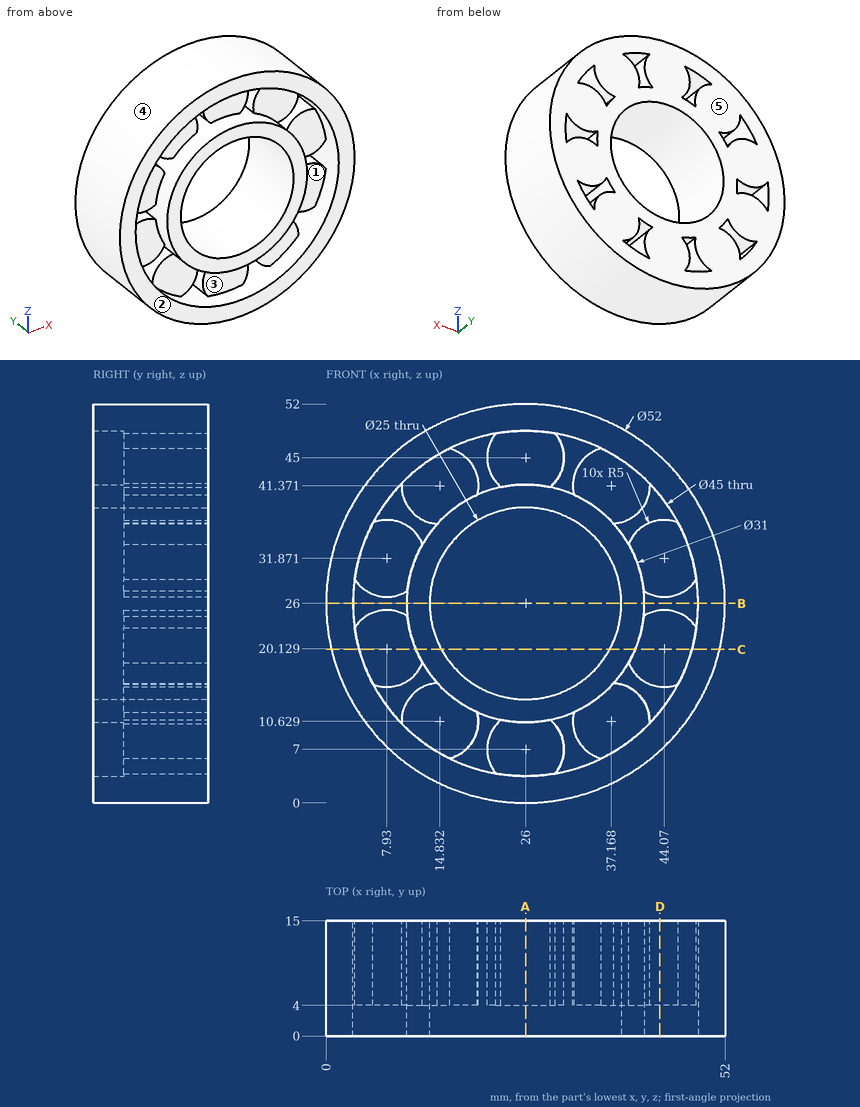
Check sheet for the drawn part. Datum: minimum x, y, z corner. Units: mm. A direction names the side the tool comes from. Give positions to 0.01 mm unless a question says otherwise; leave off trailing zeros. Order: outer loops, then holes, each group sorted by start corner. A loop starts at its lowest first (then second) coordinate and runs counter-clockwise, first axis right, second up. Notation, with made-up numbers: (13.5, 63) - (59.5, 63) arc R24 cw to (59.5, 74) - close; hole circle Ø6 at (-12, 73). An arc over 180 degrees is marked (long way). Answer in a Markdown table with one row per item. Add a question column.
Q1. Cross-section at D-D, the plane x = 43.5. Enter the section's corners in (y, z).
Q2. Mould release check, pull along X, two halves, no side actions. Record for the marked faces 3, 4 and 5: pulls with the +X half, pulls with the -X half, needs draft (parallel to the pull), parting line crosses it, or undercut.
Q3. Cross-section at B-B, the plane z = 26. Enter the section's corners in (x, y), then the cut area to 3 significant figures.
Q4. Gauge pin test, flat ends, axial feed: pin 1 (3.5 mm diameter, centred on x = 26.5, z = 5.5, fed in from -Y); pin 2 (1.5 mm diameter, centred on x = 6.5, y = 8.5, fed in from +Z); pin 3 (2 mm diameter, centred on x = 34.5, y = 12, fed in from -Z) (1 decimal). Record the tip position at first contact, or that the pin passes through.
Q5. Tool access check on the marked faces 1 and 2. Record the directions out of +Z, -Z, +X, -X, +Y, -Y that give a thin tool (end or side, any length) a straight path to the whole face; none if there is none.
Q6. Material ranges on probe 1 along Z at (x, y) = (26, 1); probe 2 along Z at (x, y) = (26, 7.25); probe 3 along X at (y, z) = (11.75, 44) (1 decimal), recorded low to high. Write a range as from..to.
Q7. Cross-section at A-A, the plane x = 26. Enter the section's corners in (y, z).
Q8. Cross-section at C-C, the plane z = 20. Enter the section's corners in (x, y) (1 decimal), then the cut area to 3 significant figures.
Check values:
| question | item | result |
|---|---|---|
| 1 | outline | (0, 6.77) - (15, 6.77) - (15, 11.86) - (0, 11.86) - close; (0, 40.14) - (15, 40.14) - (15, 45.23) - (0, 45.23) - close; (4, 15.16) - (15, 15.16) - (15, 25.1) - (4, 25.1) - close; (4, 26.9) - (15, 26.9) - (15, 36.84) - (4, 36.84) - close |
| 2 | face 3 | undercut |
| 2 | face 4 | parting line crosses it |
| 2 | face 5 | needs draft |
| 3 | outline | (0, 0) - (3.5, 0) - (3.5, 15) - (0, 15) - close; (10.5, 0) - (13.5, 0) - (13.5, 15) - (10.5, 15) - close; (38.5, 0) - (41.5, 0) - (41.5, 15) - (38.5, 15) - close; (48.5, 0) - (52, 0) - (52, 15) - (48.5, 15) - close |
| 3 | area | 195 mm^2 |
| 4 | pin 1 | stops at y = 4 |
| 4 | pin 2 | stops at z = 44.01 |
| 4 | pin 3 | stops at z = 1.1 |
| 5 | face 1 | -Y |
| 5 | face 2 | +Z, -Z, +X, -X, -Y |
| 6 | probe 1 | z = 0..3.5, 10.5..13.5, 38.5..41.5, 48.5..52 |
| 6 | probe 2 | z = 0..13.5, 38.5..52 |
| 6 | probe 3 | x = 7.2..19.1, 21.1..30.9, 32.9..44.8 |
| 7 | outline | (0, 0) - (15, 0) - (15, 13.5) - (0, 13.5) - (0, 10.5) - (4, 10.5) - (4, 3.5) - (0, 3.5) - close; (0, 38.5) - (15, 38.5) - (15, 52) - (0, 52) - (0, 48.5) - (4, 48.5) - (4, 41.5) - (0, 41.5) - close |
| 8 | outline | (0.7, 0) - (4.3, 0) - (4.3, 4) - (11.7, 4) - (11.7, 0) - (15, 0) - (15, 15) - (0.7, 15) - close; (37, 0) - (40.3, 0) - (40.3, 4) - (47.7, 4) - (47.7, 0) - (51.3, 0) - (51.3, 15) - (37, 15) - close |
| 8 | area | 371 mm^2 |
